```python
from build123d import *

# Parameters (mm, degrees)
SKETCH001_R             = 0.6
PAD004_DEPTH            = 2.8
FILLET_R                = 0.4
FILLET001_R             = 5
BODY014_PLACEMENT_ANGLE = 180


with BuildPart() as part:
    # Sketch001 (on DatumPlane) → Pad004 (new body)
    with BuildSketch(Plane(origin=(-24.3, 0, 0), x_dir=(0, -1, 0), z_dir=(-1, 0, 0))):
        Polygon((-10, 84), (10, 84), (10, -53), (6, -53), (6, -50.2), (1.25, -50.2), (1.25, -47.2), (2.75, -47.2), (2.75, -44.7), (1.25, -44.7), (1.25, -40.7), (-1.25, -40.7), (-1.25, -44.7), (-2.75, -44.7), (-2.75, -47.2), (-1.25, -47.2), (-1.25, -50.2), (-6, -50.2), (-6, -53), (-10, -53), align=None)
        with Locations((-7, 20)):
            Circle(SKETCH001_R, mode=Mode.SUBTRACT)
        with Locations((7, 20)):
            Circle(SKETCH001_R, mode=Mode.SUBTRACT)
        Polygon((1.6, -9.07624), (0, -8.152479), (-1.6, -9.07624), (-1.6, -10.92376), (0, -11.847521), (1.6, -10.92376), align=None, mode=Mode.SUBTRACT)
        with BuildLine():
            ThreePointArc((3.1, 75), (0, 78.1), (-3.1, 75))
            Line((-3.1, 75), (-3.1, 50))
            ThreePointArc((-3.1, 50), (0, 46.9), (3.1, 50))
            Line((3.1, 50), (3.1, 75))
        make_face(mode=Mode.SUBTRACT)
    extrude(amount=PAD004_DEPTH)

    # Fillet
    fillet_edges = [part.edges().sort_by_distance(p)[0] for p in [
        (-25.7, 10, -53),
        (-25.7, 6, -53),
        (-25.7, -10, -53),
        (-25.7, -6, -53),
        (-25.7, 1.25, -50.2),
        (-25.7, -1.25, -50.2),
        (-25.7, 1.25, -40.7),
        (-25.7, -1.25, -40.7),
        (-25.7, 1.25, -47.2),
        (-25.7, -1.25, -47.2),
        (-25.7, 1.25, -44.7),
        (-25.7, -1.25, -44.7),
        (-25.7, -2.75, -47.2),
        (-25.7, 2.75, -47.2),
        (-25.7, 2.75, -44.7),
        (-25.7, -2.75, -44.7),
    ]]
    fillet(fillet_edges, radius=FILLET_R)

    # Fillet001
    fillet001_edges = [part.edges().sort_by_distance(p)[0] for p in [
        (-25.7, 10, 84),
        (-25.7, -10, 84),
    ]]
    fillet(fillet001_edges, radius=FILLET001_R)


with BuildPart() as part_1:
    # Body014 placement: moved
    add(part.part.moved(Location((0, 0, 20))).rotate(Axis((0, 0, 20), (0, 0, 1)), BODY014_PLACEMENT_ANGLE))


solid = part_1.part
```
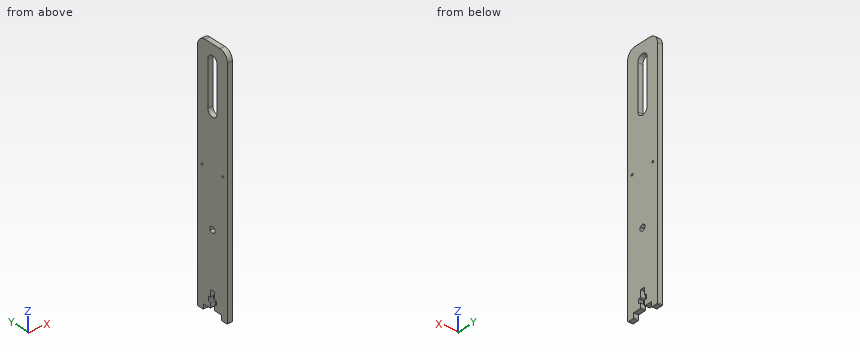
The listing builds one solid part. Answer for the finished solid, in the listing's coordinates (mm). Round coordinates to 2 decimals unless told otherwise and drop trailing zeros. Write each loop counter-clockwise with the first axis right and the second up, starting at its lowest first coordinate (ties: lowest second). Pieces come first, ordered by that corner, then holes. Notation, with made-up numbers: (22, 77.5) -> (28, 77.5) arc R23 cw to (28, 112.5) -> close; hole circle Ø3 at (-15, 2). An arc over 180 degrees is marked (long way). Answer as a JSON object with one key per item and string values. Group by question number.
Q1. Straight lines are drawn through the part: line 1 along Y through (x, z) = (25.1, 40); line 2 along Y through (x, z) = (26.4, 94.5); line 3 along Y through (x, z) = (25.45, 9). For each, find the intervals that lie inside material, in ascending order.
Q2. Section B-B (x = 26.55) is taken. Count the separate pieces of the cut face and the enclosed holes in it, plus the area to 3 significant figures.
Q3. Section A-A (z = 72) is taken. Write down the section's boundary in (x, y).
Q4. Each of these flat-tipped pins is pushed along its axis until it touches: pin 1 Ø0.9 at (x, y) = (25, 0.5) entering from -Z; pin 2 Ø0.8 at (x, y) = (25.5, 2) entering from -Z. Where does it stop, or does it pass through?
Check values:
{
 "1": {"line 1": "-10 to -7.6, -6.4 to 6.4, 7.6 to 10", "line 2": "-10 to -3.1, 3.1 to 10", "line 3": "-10 to -1.47, 1.47 to 10"},
 "2": {"separate pieces": "1", "enclosed holes": "4", "area": "2,470 mm^2"},
 "3": {"outline": "(24.3, -10) -> (27.1, -10) -> (27.1, -3.1) -> (24.3, -3.1) -> close; (24.3, 3.1) -> (27.1, 3.1) -> (27.1, 10) -> (24.3, 10) -> close"},
 "4": {"pin 1": "z = -20.71", "pin 2": "z = -30.2"}
}
